Build history of the part. All positions in model axes, mm. A direction names the side the tool comes from. Round coordinates to 2 decimals unless told otherwise and drop trailing zeros. Order: outer loops, then holes, each group sorted by start corner. A loop starts at its lowest first (then second) coordinate and runs counter-clockwise, first axis right, second up. Notation, with made-up numbers: M -35,2 L 12,2 A18 ccw 12,25 Z; hole C 11.5,-32.75 d11. An arc over 180 degrees is marked long. One line per question, with ' | ' between items. Start each with the question number.
from build123d import *

# Parameters (mm, degrees)
SKETCH_R      = 30
SKETCH_R_2    = 27.725
PAD_DEPTH     = 32
SKETCH001_R   = 10
SKETCH001_R_2 = 7.5
PAD001_DEPTH  = 3
SKETCH002_R   = 24.25
POCKET_DEPTH  = 35.001
SKETCH003_R   = 30
SKETCH003_R_2 = 23.79
PAD002_DEPTH  = 10


with BuildPart() as part:
    # Sketch → Pad (new body)
    with BuildSketch(Plane.XY):
        Circle(SKETCH_R)
        Circle(SKETCH_R_2, mode=Mode.SUBTRACT)
    extrude(amount=PAD_DEPTH)

    # Sketch001 (on Face4 of Pad) → Pad001 (join)
    with BuildSketch(Plane.XY.offset(32)):
        with BuildLine():
            ThreePointArc((-3.2, 36), (0, 32.8), (3.2, 36))
            Line((3.2, 50), (3.2, 36))
            Line((50, 50), (3.2, 50))
            Line((50, -130), (50, 50))
            Line((-50, -130), (50, -130))
            Line((-50, 50), (-50, -130))
            Line((-3.2, 50), (-50, 50))
            Line((-3.2, 50), (-3.2, 36))
        make_face()
        with Locations((0, -50.8)):
            Circle(SKETCH001_R, mode=Mode.SUBTRACT)
        with Locations((-38.1, -50.8)):
            Circle(SKETCH001_R, mode=Mode.SUBTRACT)
        with Locations((38.1, -50.8)):
            Circle(SKETCH001_R, mode=Mode.SUBTRACT)
        with Locations((-25.4, -76.2)):
            Circle(SKETCH001_R, mode=Mode.SUBTRACT)
        with Locations((25.4, -76.2)):
            Circle(SKETCH001_R, mode=Mode.SUBTRACT)
        with Locations((0, -88.9)):
            Circle(SKETCH001_R, mode=Mode.SUBTRACT)
        with Locations((-38.1, -101.6)):
            Circle(SKETCH001_R, mode=Mode.SUBTRACT)
        with Locations((38.1, -101.6)):
            Circle(SKETCH001_R, mode=Mode.SUBTRACT)
        with Locations((-12.7, -114.3)):
            Circle(SKETCH001_R, mode=Mode.SUBTRACT)
        with Locations((12.7, -114.3)):
            Circle(SKETCH001_R, mode=Mode.SUBTRACT)
        with Locations((-38.1, 38.1)):
            Circle(SKETCH001_R_2, mode=Mode.SUBTRACT)
        with Locations((38.1, 38.1)):
            Circle(SKETCH001_R_2, mode=Mode.SUBTRACT)
        with Locations((38.1, -25.4)):
            Circle(SKETCH001_R_2, mode=Mode.SUBTRACT)
        with Locations((-38.1, -25.4)):
            Circle(SKETCH001_R_2, mode=Mode.SUBTRACT)
    extrude(amount=PAD001_DEPTH)

    # Sketch002 → Pocket (cut, through all)
    with BuildSketch(Plane.XY):
        Circle(SKETCH002_R)
    extrude(amount=POCKET_DEPTH, mode=Mode.SUBTRACT)

    # Sketch003 → Pad002 (join)
    with BuildSketch(Plane.XY.offset(34)):
        Circle(SKETCH003_R)
        Circle(SKETCH003_R_2, mode=Mode.SUBTRACT)
    extrude(amount=-PAD002_DEPTH)


solid = part.part
Item 1: Flat gauge pins, fed straight in: pin 1 (13.5 mm diameter, centred on x = -38.1, y = -25.4, fed in from +Z); pin 2 (10 mm diameter, centred on x = 10.5, y = -20, fed in from +Z); pin 3 (1 mm diameter, centred on x = -16, y = -101.5, fed in from -Z); pin 4 (12 mm diameter, centred on x = -12.5, z = 18, fed in from +Y). Where does each tip first touch, or does it go through?
Item 2: Tool access for faces 4 (the face through (-0.1, 32.8, 33.5)), 5 (the face through (11.19, -21.514, 34.493)), 6 (the face through (1, -39, 32)): list every direction of +Z, -Z, +X, -X, +Y, -Y with a clear straight run to the whole face (end or side of a thin tool).
Item 3: Cut at A-A on y = -88.9. Write the cut outline in (x, z), then the cut area to 3 significant figures.
Item 4: Cut at D-D on x = -38.1. Write the cut outline in (y, z), then the cut area to 3 significant figures.
Item 5: Wall check: line 1 along Y through (x, z) = (38.1, 34.2); line 2 along X through (y, z) = (38, 33); line 3 along Y through (x, z) = (-12.7, 33.2). Give the ranges that are in metal, low to high. Write a range as [from, to].
Item 6: Cut at B-B on x = 0. Write the cut outline in (y, z) (3 decimals).
Item 7: Cut at C-C on y = 38.1. Write the cut outline in (x, z), then the cut area to 3 significant figures.
Item 8: Two-plate mould, pull along X, no slides. Class faces 1 (the face through (-29.97, 1.32, 15.78)), 2 (the face through (1, -39, 35)), 3 (the face through (-1.302, -40.885, 33.479)): +X half, -X half, draft (parallel to the pull), parting line (faces both ways), or undercut.
Results found:
1) pin 1: passes through | pin 2: stops at z = 35 | pin 3: stops at z = 32 | pin 4: stops at y = 29.29
2) face 4: +Z, -Z, +Y | face 5: +Z | face 6: -Z
3) outline: M -50,32 L -10,32 L -10,35 L -50,35 Z; M 10,32 L 50,32 L 50,35 L 10,35 Z | area: 240 mm^2
4) outline: M -130,32 L -111.6,32 L -111.6,35 L -130,35 Z; M -91.6,32 L -60.8,32 L -60.8,35 L -91.6,35 Z; M -40.8,32 L -32.9,32 L -32.9,35 L -40.8,35 Z; M -17.9,32 L 30.6,32 L 30.6,35 L -17.9,35 Z; M 45.6,32 L 50,32 L 50,35 L 45.6,35 Z | area: 330 mm^2
5) line 1: y = [-130, -111.6], [-91.6, -60.8], [-40.8, -32.9], [-17.9, 30.6], [45.6, 50] | line 2: x = [-50, -45.6], [-30.6, -3.2], [3.2, 30.6], [45.6, 50] | line 3: y = [-130, -124.3], [-104.3, -20.12], [20.12, 50]
6) outline: M -130,32 L -98.9,32 L -98.9,35 L -130,35 Z; M -78.9,32 L -60.8,32 L -60.8,35 L -78.9,35 Z; M -40.8,32 L -30,32 L -30,0 L -27.725,0 L -27.725,24 L -23.79,24 L -23.79,34 L -24.25,34 L -24.25,35 L -40.8,35 Z; M 23.79,24 L 27.725,24 L 27.725,0 L 30,0 L 30,32 L 32.8,32 L 32.8,35 L 24.25,35 L 24.25,34 L 23.79,34 Z
7) outline: M -50,32 L -45.6,32 L -45.6,35 L -50,35 Z; M -30.6,32 L -3.2,32 L -3.2,35 L -30.6,35 Z; M 3.2,32 L 30.6,32 L 30.6,35 L 3.2,35 Z; M 45.6,32 L 50,32 L 50,35 L 45.6,35 Z | area: 191 mm^2
8) face 1: parting line | face 2: draft | face 3: undercut
